Design review of the part built by this model. Coordinates are the model's own, in mm. A direction names the side the tool comes from. Give positions to 0.01 mm unless a question says otherwise; leave off trailing zeros. Loops run counter-clockwise (first coordinate to the right, second up) from the corner with the lowest first, then second, coordinate; pieces in that order, holes last. Notation, with made-up numbers: (41.25, -20.75) - (90.25, -20.75) arc R23 ccw to (90.25, -7.75) - close; hole circle Ø7 at (3.25, -20.5). An arc over 180 degrees is marked (long way). Write each question's results on one line, items separated by ' | '.
```python
from build123d import *

# Parameters (mm, degrees)
F3_R     = 2.5
F5_DEPTH = 25
F6_R     = 14.5
F6_R_2   = 13
F7_DEPTH = 68
F8_R     = 13
F9_DEPTH = 68
F10_R    = 3


with BuildPart() as f1:
    # F0 (on Front) → F1 (revolve)
    with BuildSketch(Plane.XZ):
        Polygon((-401, 13), (0, 13), (0, 14.5), (-2.255578215, 14.5), (-16.97050035, 30.7946223766), (-23, 30.7946223766), (-23, 35), (-401, 35), (-401, 56), (-421, 56), (-421, 0), (-401, 0), align=None)
    revolve(axis=Axis((-210.5, 0, 0), (-1, 0, 0)))

    # F4: sweep along a path in F2
    with BuildLine(Plane.XZ) as f4_path:
        Line((-421, 32.5), (-426, 32.5))
        ThreePointArc((-426, 32.5), (-436.6066017178, 28.1066017178), (-441, 17.5))
        Line((-441, 17.5), (-441, 0))
        Line((-441, 0), (-441, -17.5))
        ThreePointArc((-441, -17.5), (-436.6066017178, -28.1066017178), (-426, -32.5))
        Line((-426, -32.5), (-421, -32.5))
    # F3 (on face) → F4 (sweep)
    with BuildSketch(Plane(origin=(-421, 0, 0), x_dir=(0, -1, 0), z_dir=(-1, 0, 0))):
        with Locations((0, 32.5)):
            Circle(F3_R)
    sweep(path=f4_path.line)

    # F3 (on face) → F5 (cut)
    with BuildSketch(Plane(origin=(-421, 0, 0), x_dir=(0, -1, 0), z_dir=(-1, 0, 0))):
        with BuildLine():
            ThreePointArc((-3.8461538462, 49.8518515262), (0, 50), (3.8461538462, 49.8518515262))
            Line((3.8461538462, 49.8518515262), (4.3076923077, 55.8340737094))
            ThreePointArc((4.3076923077, 55.8340737094), (0, 56), (-4.3076923077, 55.8340737094))
            Line((-4.3076923077, 55.8340737094), (-3.8461538462, 49.8518515262))
        make_face()
        with BuildLine():
            ThreePointArc((50.5075723829, 24.1864658845), (48.4974226119, 28), (46.1998800752, 31.6476078248))
            Line((46.1998800752, 31.6476078248), (41.2498929243, 28.2567927007))
            ThreePointArc((41.2498929243, 28.2567927007), (43.3012701892, 25), (45.0960467705, 21.5950588255))
            Line((45.0960467705, 21.5950588255), (50.5075723829, 24.1864658845))
        make_face()
        with BuildLine():
            ThreePointArc((46.1998800752, -31.6476078248), (48.4974226119, -28), (50.5075723829, -24.1864658845))
            Line((50.5075723829, -24.1864658845), (45.0960467705, -21.5950588255))
            ThreePointArc((45.0960467705, -21.5950588255), (43.3012701892, -25), (41.2498929243, -28.2567927007))
            Line((41.2498929243, -28.2567927007), (46.1998800752, -31.6476078248))
        make_face()
        with BuildLine():
            Line((-3.8461538462, -49.8518515262), (-4.3076923077, -55.8340737094))
            ThreePointArc((-4.3076923077, -55.8340737094), (0, -56), (4.3076923077, -55.8340737094))
            Line((4.3076923077, -55.8340737094), (3.8461538462, -49.8518515262))
            ThreePointArc((3.8461538462, -49.8518515262), (0, -50), (-3.8461538462, -49.8518515262))
        make_face()
        with BuildLine():
            Line((-45.0960467705, -21.5950588255), (-50.5075723829, -24.1864658845))
            ThreePointArc((-50.5075723829, -24.1864658845), (-48.4974226119, -28), (-46.1998800752, -31.6476078248))
            Line((-46.1998800752, -31.6476078248), (-41.2498929243, -28.2567927007))
            ThreePointArc((-41.2498929243, -28.2567927007), (-43.3012701892, -25), (-45.0960467705, -21.5950588255))
        make_face()
        with BuildLine():
            Line((-41.2498929243, 28.2567927007), (-46.1998800752, 31.6476078248))
            ThreePointArc((-46.1998800752, 31.6476078248), (-48.4974226119, 28), (-50.5075723829, 24.1864658845))
            Line((-50.5075723829, 24.1864658845), (-45.0960467705, 21.5950588255))
            ThreePointArc((-45.0960467705, 21.5950588255), (-43.3012701892, 25), (-41.2498929243, 28.2567927007))
        make_face()
    extrude(amount=-F5_DEPTH, mode=Mode.SUBTRACT)

    # F6 (on Front) → F7 (join)
    with BuildSketch(Plane.XZ):
        with Locations((-320, 0)):
            Circle(F6_R)
        with Locations((-320, 0)):
            Circle(F6_R_2, mode=Mode.SUBTRACT)
    extrude(amount=F7_DEPTH)

    # F8 (on face) → F9 (cut)
    with BuildSketch(Plane.XZ.offset(68)):
        with Locations((-320, 0)):
            Circle(F8_R)
    extrude(amount=-F9_DEPTH, mode=Mode.SUBTRACT)

    # F10
    f10_edges = [f1.edges().sort_by_distance(p)[0] for p in [
        (-334.5, -35, 0),
    ]]
    fillet(f10_edges, radius=F10_R)


solid = f1.part
```
Item 1: Tool access review of faces 4 (the face through (-20.03, -30.06, -6.68)), 5 (the face through (-411, 56, 0)), 6 (the face through (-306.17, -50.63, 4.36)), 7 (the face through (-411, 0, -50)), 8 (the face through (-401, 26, -24)): name each direction out of +Z, -Z, +X, -X, +Y, -Y from which nothing blocks a thin tool from reaching the whole face with its end or side.
Output values:
face 4: +X | face 5: +X, -X, +Y | face 6: -Y | face 7: -Z, +X, -X | face 8: none
Item 2: We need section B-B on x = -48. Give the boundary of the cut face in (y, z).
Output values:
outline: circle Ø70 at (0, 0); hole circle Ø26 at (0, 0)
Item 3: Clearance check with flat-ended pins moving along their axes: P1, Ø5, axis at y = 19.5, z = 16, coming from the +X side; P2, Ø2, axis at y = -3, z = -41.5, coming from the +X side; P3, Ø11.5, axis at x = -329.5, z = -5, coming from the +Y side. State where each tip first meets the part, or that it passes through.
Output values:
P1: stops at x = -9.68 | P2: stops at x = -401 | P3: stops at y = 35
Item 4: We need section C-C on x = -407. Give the boundary of the cut face in (y, z), then the cut area to 3 significant figures.
Output values:
outline: (-50.51, -24.19) - (-45.1, -21.6) arc R50 ccw to (-41.25, -28.26) - (-46.2, -31.65) arc R56 ccw to (-4.31, -55.83) - (-3.85, -49.85) arc R50 ccw to (3.85, -49.85) - (4.31, -55.83) arc R56 ccw to (46.2, -31.65) - (41.25, -28.26) arc R50 ccw to (45.1, -21.6) - (50.51, -24.19) arc R56 ccw to (50.51, 24.19) - (45.1, 21.6) arc R50 ccw to (41.25, 28.26) - (46.2, 31.65) arc R56 ccw to (4.31, 55.83) - (3.85, 49.85) arc R50 ccw to (-3.85, 49.85) - (-4.31, 55.83) arc R56 ccw to (-46.2, 31.65) - (-41.25, 28.26) arc R50 ccw to (-45.1, 21.6) - (-50.51, 24.19) arc R56 ccw to start | area: 9,560 mm²
Item 5: Draft analysis for pull direction X (two halves, no side actions). For faces 1 (the face through (-401, 0, 0)), 2 (the face through (-411.14, 27.7, 48.67)), 3 (the face through (-23, -31, 0)), state which applies: +X half, -X half, draft (parallel to the pull), parting line (faces both ways), or undercut.
Output values:
face 1: undercut | face 2: draft | face 3: +X half
Item 6: Wall thickness on probe 1 along Z at (x, y) = (-320, -54); probe 2 along X at (y, z) = (-28, 0); probe 3 along Y at (x, z) = (-251, -18): over which ranges is each line inside the solid? List them lowest first.
Output values:
probe 1: z = -14.5 to -13, 13 to 14.5 | probe 2: x = -421 to -333, -307 to -14.45 | probe 3: y = -30.02 to 30.02
Item 7: We need section A-A on z = 0. Give the number of separate pieces and of enclosed holes in the cut face, then the cut area to 3 significant figures.
Output values:
separate pieces: 3 | enclosed holes: 0 | area: 19,000 mm²
